Autodesk Inventor part; units mm, degrees
ref_plane "YZ Plane" through (0, 0, 0) normal (1, 0, 0) x (0, 1, 0)
ref_plane "XZ Plane" through (0, 0, 0) normal (0, 1, 0) x (-1, 0, 0)
ref_plane "XY Plane" through (0, 0, 0) normal (0, 0, 1) x (1, 0, 0)
sketch "Sketch1" plane through (0, 0, 0) normal (1, 0, 0) x (0, 1, 0)
  line L0 (10.5, 12) -> (-10.5, 12)
  line L1 (-10.5, 12) -> (-10.5, -12)
  line L2 (-10.5, -12) -> (10.5, -12)
  line L3 (10.5, -12) -> (10.5, 12)
  line L4 (10.5, 12) -> (-10.5, -12) construction
  line L5 (-10.5, 12) -> (10.5, -12) construction
  point P0 (0, 0)
  dimension "d0" = 21
  dimension "d1" = 24
extrude "Extrusion1" add sketch "Sketch1" along normal mid plane 11.6
sketch "Sketch2" plane through (5.8, 0, 0) normal (1, 0, 0) x (0, 0, -1)
  line L0 (-12, 9.5) -> (-16.4, 9.5)
  line L1 (-16.4, 9.5) -> (-16.4, 7.58)
  line L2 (-16.4, 7.58) -> (-12, 7.58)
  line L3 (-12, 7.58) -> (-12, 9.5)
  line L4 (-12, -10.5) -> (12, -10.5)
  line L5 (0, -10.5) -> (0, 10.5)
  line L6 (12, 9.5) -> (16.4, 9.5)
  line L7 (16.4, 9.5) -> (16.4, 7.58)
  line L8 (16.4, 7.58) -> (12, 7.58)
  line L9 (12, 7.58) -> (12, 9.5)
  line L10 (-12, 9.5) -> (-13.7444, 9.5)
  point P0 (0, 0)
  point P1 (-12, 10.5)
  dimension "d4" = 4.4
  dimension "d5" = 1.92
  dimension "d8" = 1
extrude "Extrusion2" add sketch "Sketch2" against normal up to surface (11.6 mm away)
sketch "Sketch3" plane through (5.8, 0, 0) normal (1, 0, 0) x (0, 0, -1)
  line L0 (-12, 10.5) -> (3, 10.5)
  line L1 (3, 10.5) -> (3, 16.6)
  line L2 (3, 16.6) -> (-12, 16.6)
  line L3 (-12, 16.6) -> (-12, 10.5)
  line L4 (12, 10.5) -> (-12, 10.5)
  point P0 (0, 0)
  dimension "d9" = 15
  dimension "d10" = 6.1
extrude "Extrusion3" add sketch "Sketch3" against normal up to surface (11.6 mm away)
sketch "Sketch4" plane through (5.8, 16.6, 12) normal (0, 1, 0) x (1, 0, 0)
  circle A0 centre (-5.8, 6.9504) radius 2.829
  point P0 (-5.8, 12)
extrude "Extrusion4" add sketch "Sketch4" along normal blind 2
properties part number "servoMotor"
Input: part model. Units: mm. Frame: model coordinates. A direction names the side the tool comes from. Coordinates: 2 decimals unless noted, no trailing zeros. Loops run counter-clockwise (first coordinate to the right, second up) from the corner with the lowest first, then second, coordinate; pieces in that order, holes last. Notation, with made-up numbers: M 64,66.5 L 84,66.5 A28 ccw 84,84.5 Z; hole C 48.25,15.25 d3. An arc over 180 degrees is marked long. One line per item, written item: value.
(1) Section D-D (x = -3.5). Output: boundary loops of the cut face in (y, z).
Filled in:
outline: M -10.5,-12 L 7.58,-12 L 7.58,-16.4 L 9.5,-16.4 L 9.5,-12 L 10.5,-12 L 10.5,-3 L 16.6,-3 L 16.6,12 L 9.5,12 L 9.5,16.4 L 7.58,16.4 L 7.58,12 L -10.5,12 Z
(2) Reachability of faces 1 (the flat face through (0, 13, 12)), 2 (the flat face through (0, -2, -12)), 3 (the flat face through (0, 10, -12)), 4 (the flat face through (3, 16.6, 3)) from +Z, -Z, +X, -X, +Y, -Y: full face, straight path, thin tool, end or side. Return the list, or none.
Filled in:
face 1: +Z, +X, -X, +Y
face 2: -Z, +X, -X, -Y
face 3: -Z, +X, -X, +Y
face 4: +Y
(3) Line query: line 1 along Y through (x, z) = (0.5, 15); line 2 along Y through (x, z) = (-1.75, -2); line 3 along Z through (x, y) = (3.25, 1). Output: solid intervals per line, ascending. Write a range as from..to.
Filled in:
line 1: 7.58..9.5
line 2: -10.5..16.6
line 3: -12..12
(4) Section C-C (z = 4). Output: boundary loops of the cut face in (x, y).
Filled in:
outline: M -5.8,-10.5 L 5.8,-10.5 L 5.8,16.6 L 2.63,16.6 L 2.63,18.6 L -2.63,18.6 L -2.63,16.6 L -5.8,16.6 Z
(5) Section B-B (y = 15.5). Output: boundary loops of the cut face in (x, z).
Filled in:
outline: M -5.8,-3 L 5.8,-3 L 5.8,12 L -5.8,12 Z
(6) Section A-A (x = 0). Output: boundary loops of the cut face in (y, z), and give its area (3 significant figures).
Filled in:
outline: M -10.5,-12 L 7.58,-12 L 7.58,-16.4 L 9.5,-16.4 L 9.5,-12 L 10.5,-12 L 10.5,-3 L 16.6,-3 L 16.6,2.22 L 18.6,2.22 L 18.6,7.88 L 16.6,7.88 L 16.6,12 L 9.5,12 L 9.5,16.4 L 7.58,16.4 L 7.58,12 L -10.5,12 Z
area: 624 mm^2
(7) Pin query (flat end, axial travel): pin 1 (2 mm diameter, centred on x = -1, y = 13.5, fed in from +Z); pin 2 (2 mm diameter, centred on x = -2, z = 13.5, fed in from +Y); pin 3 (3.5 mm diameter, centred on x = 3, z = -13.5, fed in from -Y); pin 4 (1.5 mm diameter, centred on x = -4, y = 12.5, fed in from -Z). Return the tip coordinate at first contact, or that it passes through.
Filled in:
pin 1: z = 12
pin 2: y = 9.5
pin 3: y = -10.5
pin 4: z = -3
